The model under review builds one solid part; all positions refer to its coordinate system, in mm. Face numbers are marked on the shaded views. A direction names the side the tool comes from. Coordinates: 2 decimals unless noted, no trailing zeros. Write each loop counter-clockwise with the first axis right and the second up, starting at its lowest first coordinate (ties: lowest second). Pieces come first, ordered by that corner, then holes.
1) Machinability: for the marked faces 1 and 2, which of the approach directions +Z, -Z, +X, -X, +Y, -Y give a long, thin tool a straight path to every point of the face, cutting with its end or side? Answer none if there is none.
2) Add section C-C, the plane z = 54. State the section outline as (x, y) points, then the cut area to 3 significant figures.
3) Mouldability with a two-part tool opening along X and no side actions: class the marked faces 3, 4 and 5 as released by +X, released by -X, zero draft, split by the parting line, or undercut.
4) Add section D-D, the plane z = 18.5. State the section outline as (x, y) points.
5) Add section A-A, the plane x = -41.5. State the section outline as (y, z) points.
6) For line 1 (X direction, y = -37, z = 50); line 2 (Y direction, x = 20, z = 31.5); line 3 (X direction, y = -21, z = 47), list the stretches that pass through material, from the lowest coordinate up.
7) For P1, Ø4, axis at x = 21, y = -22, coming from the +Z side; P2, Ø20.5, axis at y = -41.5, z = 34.5, coming from the +X side; P3, Ø7.5, axis at x = 9, y = -42, coming from the +Z side, all flat-tipped, find the tip position at first contact; note any pin that passes through.
8) Add section B-B, the plane y = -34.5. State the section outline as (x, z) points.
from build123d import *

# Parameters (mm, degrees)
F0_R     = 12.7
F1_DEPTH = 25.4
F2_R     = 12.7
F3_DEPTH = 25.4
F4_R     = 12.7


with BuildPart() as f1:
    # F0 (on Front) → F1 (new body)
    with BuildSketch(Plane.XZ):
        with BuildLine():
            Line((61.112298, 12.7), (-26.23751, 71.838392))
            ThreePointArc((-26.23751, 71.838392), (-52.389372, 73.242992), (-65.887702, 50.8))
            Line((-65.887702, 50.8), (-65.887702, 0))
            Line((-65.887702, 0), (61.112298, 0))
            Line((61.112298, 0), (61.112298, 12.7))
        make_face()
        with Locations((-40.48112, 50.8)):
            Circle(F0_R, mode=Mode.SUBTRACT)
    extrude(amount=F1_DEPTH)

    # F2 (on face) → F3 (join)
    with BuildSketch(Plane.XZ.offset(25.4)):
        with BuildLine():
            Line((61.112298, 0), (61.112298, 12.7))
            Line((61.112298, 12.7), (-15.074539, 12.7))
            Line((-15.074539, 12.7), (-15.074539, 50.8))
            ThreePointArc((-15.074539, 50.8), (-18.038128, 62.708252), (-26.23751, 71.838392))
            ThreePointArc((-26.23751, 71.838392), (-52.389372, 73.242992), (-65.887702, 50.8))
            Line((-65.887702, 50.8), (-65.887702, 12.7))
            Line((-65.887702, 12.7), (-65.887702, 0))
            Line((-65.887702, 0), (61.112298, 0))
        make_face()
        with Locations((-40.48112, 50.8)):
            Circle(F2_R, mode=Mode.SUBTRACT)
    extrude(amount=F3_DEPTH)

    # F4
    f4_edges = [f1.edges().sort_by_distance(p)[0] for p in [
        (61.112298, -50.8, 6.35),
    ]]
    fillet(f4_edges, radius=F4_R)


solid = f1.part
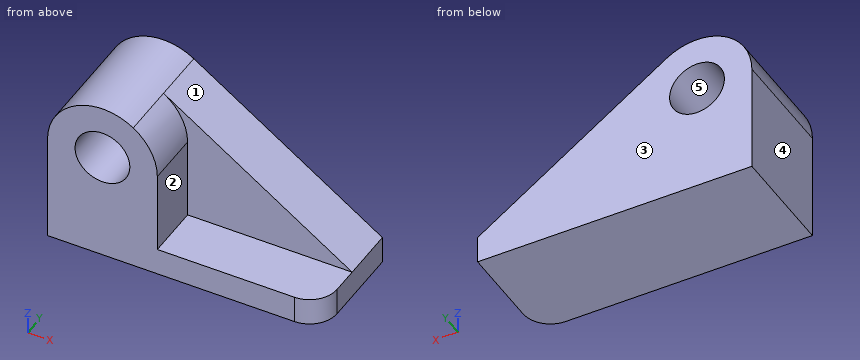
Geometry results:
1. face 1: +Z, +X, +Y, -Y
1. face 2: +Z, +X, -Y
2. outline: (-65.69, -50.8) - (-52.77, -50.8) - (-52.77, 0) - (-65.69, 0) - close; (-28.19, -50.8) - (-15.28, -50.8) - (-15.28, -25.4) - (0.11, -25.4) - (0.11, 0) - (-28.19, 0) - close
2. area: 1,700 mm2
3. face 3: zero draft
3. face 4: released by -X
3. face 5: undercut
4. outline: (-65.89, -50.8) - (-15.07, -50.8) - (-15.07, -25.4) - (52.55, -25.4) - (52.55, 0) - (-65.89, 0) - close
5. outline: (-50.8, 0) - (0, 0) - (0, 38.14) - (-50.8, 38.14) - close; (-50.8, 63.46) - (0, 63.46) - (0, 76.19) - (-50.8, 76.19) - close
6. line 1: x = -65.89 to -53.16, -27.81 to -15.07
6. line 2: y = -25.4 to 0
6. line 3: x = -65.89 to -52.6, -28.36 to 10.45
7. P1: stops at z = 41.21
7. P2: stops at x = -15.07
7. P3: stops at z = 12.7
8. outline: (-65.89, 0) - (61.11, 0) - (61.11, 12.7) - (-15.07, 12.7) - (-15.07, 50.8) arc R25.41 ccw to (-65.89, 50.8) - close; hole circle Ø25.4 at (-40.48, 50.8)
